from build123d import *

# Parameters (mm, degrees)
CROQUIS1_R              = 1.75
SALIENTE_EXTRUIR1_DEPTH = 3


with BuildPart() as part:
    # Croquis1 → Saliente-Extruir1 (new body)
    with BuildSketch(Plane(origin=(0, 0, 0), x_dir=(0, 0, -1), z_dir=(1, 0, 0))):
        with BuildLine():
            Line((4.703111933, 1.793661764), (-2.482700505, 21.6730463))
            Line((-2.482700505, 21.6730463), (0.053198949, 137.784671118))
            Line((0.053198949, 137.784671118), (4.5784072, 148.082410318))
            ThreePointArc((4.5784072, 148.082410318), (2.012416575, 154.671468833), (-4.57664194, 152.105478208))
            Line((-4.57664194, 152.105478208), (-7.795940026, 144.779518768))
            Line((-7.795940026, 144.779518768), (-10.634536468, 14.808259621))
            Line((-10.634536468, 14.808259621), (-4.701346672, -1.605773238))
            ThreePointArc((-4.701346672, -1.605773238), (1.700600132, -4.60828504), (4.703111933, 1.793661764))
        make_face()
        with Locations((0.00088263, 150.093944263)):
            Circle(CROQUIS1_R, mode=Mode.SUBTRACT)
        with Locations((0.00088263, 0.093944263)):
            Circle(CROQUIS1_R, mode=Mode.SUBTRACT)
    extrude(amount=SALIENTE_EXTRUIR1_DEPTH)


solid = part.part
Input: part model. Units: mm. Frame: model coordinates. A direction names the side the tool comes from. Coordinates: 2 decimals unless noted, no trailing zeros. Write each loop counter-clockwise with the first axis right and the second up, starting at its lowest first coordinate (ties: lowest second). Pieces come first, ordered by that corner, then holes. Notation, with made-up numbers: M 79,80 L 121,80 A10 cw 121,94 Z; hole C 54,64 d4. An arc over 180 degrees is marked long. Answer as a JSON object with one key per item and string values. Group by question number.
(1) Set-up query: faces 1 (the face through (1.48, 11.59, -1.16)), 2 (the face through (1.479, 148.494, 6.164)). Return all of +Z, -Z, +X, -X, +Y, -Y with unobstructed straight access to the full face (end or side cutting, diameter ignored); none if empty.
(2) Mould query, pull axis Z, two halves, no side actions, for faces 3 (the face through (1.479, 154.626, -2.113)), 4 (the face through (1.479, -1.614, 0.378)), 5 (the face through (1.5, 142.9, -2.3)), 6 (the face through (1.479, 148.386, 0.378)). Classes: pulls with the +Z half, pulls with the -Z half, needs draft (parallel to the pull), parting line crosses it, or undercut.
(3) Section B-B on y = 9.5. Output: boundary loops of the cut face in (x, z), plus the area to 3 significant figures.
(4) Section C-C on y = 134.5. Output: boundary loops of the cut face in (x, z).
(5) Ray query, line 1 along Z through (x, y) = (1.9, 14); line 2 along Z through (x, y) = (0.55, 35); line 3 along Z through (x, y) = (0.7, 149). Return the intervals inside material, ascending. Write a range as [from, to].
(6) Contact query for flat-ended pins moving along their axis: P1, Ø1.5, axis at x = 1.5, y = 22, coming from the -Z side; P2, Ø1, axis at x = 2, y = 126.5, coming from the +Z side; P3, Ø1.5, axis at y = 96, z = 0, coming from the -X side. Output: stop coordinate, or through.
(7) Section A-A on x = 2.15. Output: boundary loops of the cut face in (y, z).
Result set:
{
 "1": {"face 1": "-Z, +X, -X", "face 2": "+Z, +X, -X, +Y"},
 "2": {"face 3": "parting line crosses it", "face 4": "undercut", "face 5": "pulls with the -Z half", "face 6": "undercut"},
 "3": {"outline": "M 0,-1.92 L 3,-1.92 L 3,8.72 L 0,8.72 Z", "area": "31.9 mm2"},
 "4": {"outline": "M 0,0.02 L 3,0.02 L 3,8.02 L 0,8.02 Z"},
 "5": {"line 1": "z = [-0.29, 10.34]", "line 2": "z = [2.19, 10.19]", "line 3": "z = [-4.88, -1.37], [1.37, 5.94]"},
 "6": {"P1": "stops at z = 2.33", "P2": "stops at z = 8.21", "P3": "passes through"},
 "7": {"outline": "M -1.61,4.7 A5 ccw 1.79,-4.7 L 21.67,2.48 L 137.78,-0.05 L 148.08,-4.58 A5 ccw 152.11,4.58 L 144.78,7.8 L 14.81,10.63 Z; hole C 0.09,0 d3.5; hole C 150.09,0 d3.5"}
}
